Autodesk Inventor part; units mm, degrees
ref_plane "YZ Plane" through (0, 0, 0) normal (1, 0, 0) x (0, 1, 0)
ref_plane "XZ Plane" through (0, 0, 0) normal (0, 1, 0) x (-1, 0, 0)
ref_plane "XY Plane" through (0, 0, 0) normal (0, 0, 1) x (1, 0, 0)
sketch "Sketch1" plane through (0, 0, 0) normal (0, 1, 0) x (-1, 0, 0)
  line L0 (25, 25) -> (-25, 25)
  line L1 (-25, 25) -> (-25, -25)
  line L2 (-25, -25) -> (25, -25)
  line L3 (25, -25) -> (25, 25)
  line L4 (25, 25) -> (-25, -25) construction
  line L5 (-25, 25) -> (25, -25) construction
  point P0 (0, 0)
  dimension "d0" = 50
  dimension "d1" = 50
extrude "Extrusion1" add sketch "Sketch1" along normal blind 10
sketch "Sketch3" plane through (0, 0, 0) normal (0, 0, 1) x (1, 0, 0)
  circle A0 centre (0, 50) radius 25
  circle A1 centre (0, 50) radius 15
  line L0 (-25, 0) -> (25, 0)
  line L1 (25, 10) -> (-25, 10)
  line L2 (-25, 50) -> (-25, 10)
  line L3 (-25, 10) -> (25, 10)
  line L4 (25, 10) -> (25, 50)
  point P0 (0, 0)
  point P1 (0, 0)
  dimension "d4" = 30
  dimension "d5" = 50
  dimension "d6" = 50
extrude "Extrusion2" add sketch "Sketch3" along normal mid plane 20
properties part number "Manipulator Base"
Can you work these out from the model? Positions are in its coordinate system, mm. A direction names the side the tool comes from. Give positions to 0.01 mm unless a question says otherwise; leave off trailing zeros. Write each loop counter-clockwise with the first axis right and the second up, starting at its lowest first coordinate (ties: lowest second). Pieces come first, ordered by that corner, then holes. Notation, with made-up numbers: (14.5, -0.5) -> (21.5, -0.5) arc R26 ccw to (21.5, 29.5) -> close; hole circle Ø4 at (83.5, -16). An arc over 180 degrees is marked (long way). Answer as a JSON object with one key per item and string values. Group by question number.
Item 1: Suppose I cut it at D-D (z = 22). Please give me the cut outline in (x, y), plus the area to 3 significant figures.
Item 2: We'd pull the mould along Y, two halves only. Please class faces 1 (the face through (0, 10, 18)), 2 (the face through (-1.953, 35.128, -0.14)), 3 (the face through (-25, 19, 0)), 4 (the face through (0, 0, 0)): +Y half, -Y half, draft (parallel to the pull), parting line (faces both ways), or undercut.
Item 3: Suppose I cut it at A-A (x = 0). Please give me the cut outline in (y, z).
Item 4: Please list where these lines run through material, in increasing order: line 1 (Y direction, x = 0, z = 1.75); line 2 (Z direction, x = 3, y = 70); line 3 (Y direction, x = -10, z = -12.5). Write a range as [from, to].
Item 5: Suppose I cut it at C-C (y = 39). Please give me the cut outline in (x, z), plus the area to 3 significant figures.
Item 6: I'm going to push flat-ended pins straight in: P1, Ø12, axis at x = 4, y = 61, coming from the +Z side; P2, Ø12, axis at x = -3.5, z = 15.5, coming from the +Y side; P3, Ø1, axis at y = 63.5, z = 5, coming from the +X side. Where does each tip first touch, or does it pass through?
Item 7: Suppose I cut it at B-B (z = -2). Please give me the cut outline in (x, y), plus the area to 3 significant figures.
Item 8: For faces 5 (the face through (-6, 36, 10)), 6 (the face through (0, 5, 25)), 7 (the face through (-6, 36, -10)), which set-ups out of +Z, -Z, +X, -X, +Y, -Y let a thin tool reach every point of the face, with its end or its side?
Findings:
{
 "1": {"outline": "(-25, 0) -> (25, 0) -> (25, 10) -> (-25, 10) -> close", "area": "500 mm²"},
 "2": {"face 1": "+Y half", "face 2": "undercut", "face 3": "draft", "face 4": "-Y half"},
 "3": {"outline": "(0, -25) -> (10, -25) -> (10, -10) -> (35, -10) -> (35, 10) -> (10, 10) -> (10, 25) -> (0, 25) -> close; (65, -10) -> (75, -10) -> (75, 10) -> (65, 10) -> close"},
 "4": {"line 1": "y = [0, 35], [65, 75]", "line 2": "z = [-10, 10]", "line 3": "y = [0, 10]"},
 "5": {"outline": "(-25, -10) -> (-10.2, -10) -> (-10.2, 10) -> (-25, 10) -> close; (10.2, -10) -> (25, -10) -> (25, 10) -> (10.2, 10) -> close", "area": "592 mm²"},
 "6": {"P1": "stops at z = 10", "P2": "stops at y = 74.98", "P3": "stops at x = 21.35"},
 "7": {"outline": "(-25, 0) -> (25, 0) -> (25, 50) arc R25 ccw to (-25, 50) -> close; hole circle Ø30 at (0, 50)", "area": "2,770 mm²"},
 "8": {"face 5": "+Z, +X, -X, +Y", "face 6": "+Z, +X, -X, +Y, -Y", "face 7": "-Z, +X, -X, +Y"}
}
